Read the model definition and answer for the solid it produces. Units are mm, in the model's axes. A direction names the side the tool comes from. Round coordinates to 2 decimals unless told otherwise and drop trailing zeros. Order: outer loops, then holes, each group sorted by start corner. A loop starts at its lowest first (then second) coordinate and runs counter-clockwise, first axis right, second up. Notation, with made-up numbers: (71, 60.5) - (107, 60.5) arc R24 ccw to (107, 88.5) - close; hole circle Ø1 at (73.25, 37). An arc over 180 degrees is marked (long way). One line per question, with ' | ' between items. Start each with the question number.
1) The part is cut by section A-A, the plane z = 1.25. Give the vertices of the cut face in (x, y), plus the area to 3 significant figures.
2) Straight lines are drawn through the part: line 1 (X direction, y = 17, z = 1.05); line 2 (X direction, y = 8.5, z = 1.85); line 3 (Y direction, x = -4.5, z = 0.95). For each, find the intervals that lie inside material, in ascending order. Write a range as from..to.
3) Flat-ended cylindrical pins translate along their axes: pin 1 (10 mm diameter, centred on x = 139.5, y = 17.5, fed in from -Z); pin 2 (1 mm diameter, centred on x = 110, z = 1.5, fed in from -Y); pin 3 (2 mm diameter, centred on y = -15, z = 3.5, fed in from +X). Find the tip coordinate at first contact, or state that the pin passes through.
4) For faces 5 (the flat face through (0.914, 8.133, 2.465)), 6 (the flat face through (179.493, 9, 2.465)), 7 (the cylindrical face through (161.341, 14.987, 2.465)), determine the directions among +Z, -Z, +X, -X, +Y, -Y from which every point of the face is accessible in a straight line to the end or side of a thin tool.
5) The part is cut by section B-B, the plane x = 132. Give the vertices of the cut face in (y, z).
6) The part is cut by section C-C, the plane x = 157. Give the vertices of the cut face in (y, z), plus the area to 3 significant figures.
7) The mould has two halves that part along X. Classify faces 1 (the cylindrical face through (9.44, -20.43, 2.46)), 2 (the cylindrical face through (194.1, 21.6, 2.5)), 3 (the cylindrical face through (173.85, 22.96, 2.46)), 4 (the cylindrical face through (179.793, -16.253, 2.465)): pulls with the +X half, pulls with the -X half, needs draft (parallel to the pull), parting line crosses it, or undercut.
from build123d import *

# Parameters (mm, degrees)
BOSS_EXTRUDE1_DEPTH = 5


with BuildPart() as part:
    # Sketch1 → Boss-Extrude1 (new body)
    with BuildSketch(Plane.XY):
        with BuildLine():
            Line((7.5, 4.330127019), (7.5, -4.330127019))
            Line((7.5, -4.330127019), (0, -8.660254038))
            Line((0, -8.660254038), (-12.990381057, -1.160254038))
            ThreePointArc((-12.990381057, -1.160254038), (-10.606601718, -19.266855756), (7.5, -21.650635095))
            ThreePointArc((7.5, -21.650635095), (9.470749841, -20.408378389), (11.339164993, -19.016946938))
            ThreePointArc((11.339164993, -19.016946938), (22.116918375, -12.378980702), (34.216242145, -8.660254038))
            Line((34.216242145, -8.660254038), (143.609407991, -9.295451439))
            ThreePointArc((143.609407991, -9.295451439), (156.576488353, -10.522513679), (168.786666574, -15.057092233))
            ThreePointArc((168.786666574, -15.057092233), (179.94830651, -16.20923796), (188.786247547, -9.295451439))
            Line((188.786247547, -9.295451439), (175.79586649, -1.795451439))
            Line((175.79586649, -1.795451439), (175.79586649, 6.864802599))
            Line((175.79586649, 6.864802599), (183.29586649, 11.194929618))
            Line((183.29586649, 11.194929618), (196.286247547, 3.694929618))
            ThreePointArc((196.286247547, 3.694929618), (193.902468208, 21.801531335), (175.79586649, 24.185310674))
            ThreePointArc((175.79586649, 24.185310674), (173.82511705, 22.943054244), (171.956702255, 21.55162313))
            ThreePointArc((171.956702255, 21.55162313), (161.178948559, 14.913656483), (149.079624345, 11.194929618))
            Line((149.079624345, 11.194929618), (39.686458499, 11.830127019))
            ThreePointArc((39.686458499, 11.830127019), (26.719378137, 13.057189259), (14.509199916, 17.591767813))
            ThreePointArc((14.509199916, 17.591767813), (3.34755998, 18.74391354), (-5.490381057, 11.830127019))
            Line((-5.490381057, 11.830127019), (7.5, 4.330127019))
        make_face()
    extrude(amount=BOSS_EXTRUDE1_DEPTH)


solid = part.part
Values:
1) outline: (-12.99, -1.16) arc R15 ccw to (7.5, -21.65) arc R30 ccw to (11.34, -19.02) arc R50 cw to (34.22, -8.66) - (143.61, -9.3) arc R50 cw to (168.79, -15.06) arc R15 ccw to (188.79, -9.3) - (175.8, -1.8) - (175.8, 6.86) - (183.3, 11.19) - (196.29, 3.69) arc R15 ccw to (175.8, 24.19) arc R30 ccw to (171.96, 21.55) arc R50 cw to (149.08, 11.19) - (39.69, 11.83) arc R50 cw to (14.51, 17.59) arc R15 ccw to (-5.49, 11.83) - (7.5, 4.33) - (7.5, -4.33) - (0, -8.66) - close | area: 4,860 mm^2
2) line 1: x = -0.53..15.66, 165.28..197.13 | line 2: x = 0.28..178.63, 187.96..198.05 | line 3: y = -22.97..-6.06, 11.26..13.33
3) pin 1: passes through | pin 2: stops at y = -9.1 | pin 3: stops at x = 184.52
4) face 5: +Z, -Z, -X | face 6: +Z, -Z | face 7: +Z, -Z, +Y
5) outline: (-9.23, 0) - (11.29, 0) - (11.29, 5) - (-9.23, 5) - close
6) outline: (-10.62, 0) - (13.24, 0) - (13.24, 5) - (-10.62, 5) - close | area: 119 mm^2
7) face 1: pulls with the +X half | face 2: parting line crosses it | face 3: pulls with the -X half | face 4: undercut
